Autodesk Inventor part; units mm, degrees
ref_plane "YZ Plane" through (0, 0, 0) normal (1, 0, 0) x (0, 1, 0)
ref_plane "XZ Plane" through (0, 0, 0) normal (0, 1, 0) x (-1, 0, 0)
ref_plane "XY Plane" through (0, 0, 0) normal (0, 0, 1) x (1, 0, 0)
sketch "Sketch1" plane through (0, 0, 0) normal (0, 0, 1) x (1, 0, 0)
  line L0 (0, 12.95) -> (0, -12.95) construction
  line L1 (-21, 0) -> (21, 0) construction
  line L2 (-15, 9.25) -> (15, 9.25)
  line L3 (15, 9.25) -> (15, -9.25)
  line L4 (15, -9.25) -> (-15, -9.25)
  line L5 (-15, -9.25) -> (-15, 9.25)
  point P0 (0, 0)
  dimension "d0" = 18.5
  dimension "d1" = 30
extrude "Extrusion1" add sketch "Sketch1" along normal blind 12
sketch "Sketch2" plane through (0, 0, 0) normal (0, 0, -1) x (-1, 0, 0)
  line L0 (-15, 9.25) -> (15, -9.25) construction
  line L1 (15, 9.25) -> (-15, -9.25) construction
  point P0 (0, 0)
  point P1 (0, 0)
hole "Hole1" at (0, 0, 0) direction (0, 0, 1) diameter 3.242 end through all
sketch "Sketch3" plane through (0, 0, 12) normal (0, 0, 1) x (1, 0, 0)
  line L0 (15, 9.25) -> (15, -9.25)
  line L1 (-15, 9.25) -> (15, 9.25)
  line L2 (-15, -9.25) -> (-15, 9.25)
  line L3 (15, -9.25) -> (-15, -9.25)
  line L4 (-15, 0) -> (15, 0) construction
  line L5 (0, 9.25) -> (0, -9.25) construction
  line L6 (-11.3, 6.3) -> (11.3, 6.3) construction
  line L7 (11.3, 6.3) -> (11.3, -6.3) construction
  line L8 (11.3, -6.3) -> (-11.3, -6.3) construction
  line L9 (-11.3, -6.3) -> (-11.3, 6.3) construction
  dimension "d11" = 12.6
  dimension "d12" = 22.6
hole "Hole2" at (-11.3, 6.3, 12) at (11.3, 6.3, 12) at (11.3, -6.3, 12) at (-11.3, -6.3, 12) direction (0, 0, -1) diameter 3 depth 7
sketch "Sketch4" plane through (0, 0, 12) normal (0, 0, 1) x (1, 0, 0)
  circle A0 centre (11.3, -6.3) radius 1.5
  circle A1 centre (-11.3, 6.3) radius 1.5
  circle A2 centre (0, 0) radius 1.621
  line L0 (-11.3, 6.3) -> (11.3, 6.3)
  line L1 (11.3, 6.3) -> (11.3, -6.3)
  line L2 (11.3, -6.3) -> (-11.3, -6.3)
  line L3 (-11.3, -6.3) -> (-11.3, 6.3)
extrude "Extrusion2" cut sketch "Sketch4" against normal blind 7 contours L1 L2 A0 | A0 L2 L3 A1 L0 L1 | A1 L3 L0 picked at (10.3125, -6.1887) picked at (-10.4586, 5.7713)
sketch "Sketch5" plane through (-15, 9.25, 0) normal (0, 1, 0) x (1, 0, 0)
  line L0 (5.2, -12) -> (5.2, -5) construction
  line L1 (24.8, -12) -> (5.2, -12) construction
  line L2 (24.8, -5) -> (24.8, -12) construction
  line L3 (5.2, -5) -> (24.8, -5) construction
  line L4 (24.8, -8.5) -> (5.2, -8.5) construction
  point P0 (15, 0)
  point P1 (15, -8.5)
  dimension "d33" = 9.8
hole "Hole3" at (0, 9.25, 8.5) direction (0, -1, 0) diameter 2.459 end through all
sketch "Sketch6" plane through (-15, 9.25, 0) normal (0, 1, 0) x (1, 0, 0)
  line L0 (0, 0) -> (30, 0)
  line L1 (15, 2.4) -> (15, -14.4) construction
  line L2 (2.5, 0) -> (27.5, 0)
  line L3 (27.5, 0) -> (27.5, -2)
  line L4 (27.5, -2) -> (2.5, -2)
  line L5 (2.5, -2) -> (2.5, 0)
  point P0 (15, 0)
  dimension "d29" = 25
  dimension "d30" = 2
extrude "Extrusion3" cut sketch "Sketch6" against normal up to next
properties part number "Küvettenklammer_20mm_version3"
Geometry: final body of the model. Coordinates: model frame, mm. A direction names the side the tool comes from. Round coordinates to 2 decimals unless told otherwise and drop trailing zeros. Write each loop counter-clockwise with the first axis right and the second up, starting at its lowest first coordinate (ties: lowest second). Pieces come first, ordered by that corner, then holes.
Item 1: Mould query, pull axis X, two halves, no side actions, for faces 4 (the face through (15, 0, 6)), 5 (the face through (-0.369, -7.796, 9.673)), 6 (the face through (0, -9.25, 7)). Classes: +X half, -X half, draft (parallel to the pull), parting line (faces both ways), or undercut.
Item 2: Material intervals for L1, parallel to Z at x = 0, y = -7.15; L2, parallel to Y at x = 0, z = 3.3; L3, parallel to Y at x = 1.5, z = 10.75, sorted ascending.
Item 3: Section query B-B (y = 0). Return loops of the section in (x, z), plus the area to 3 significant figures.
Item 4: Section query A-A (x = 0). Return loops of the section in (y, z), plus the area to 3 significant figures.
Item 5: Section query C-C (z = 8.5). Return loops of the section in (x, y).
Item 6: Pin query (flat end, axial travel): P1, Ø5, axis at x = 0, y = 0, coming from the -Z side; P2, Ø2, axis at x = 0, z = 8.5, coming from the +Y side; P3, Ø4.5, axis at x = 5.5, y = -1.5, coming from the +Z side. Return the tip coordinate at first contact, or that it passes through.
Item 7: Set-up query: faces 1 (the face through (12.5, 0, 1)), 2 (the face through (1.438, 0.748, 3.521)), 3 (the face through (-11.3, 0, 9)). Return all of +Z, -Z, +X, -X, +Y, -Y with unobstructed straight access to the full face (end or side cutting, diameter ignored); none if empty.
Item 8: Section query D-D (y = -7.5). Return loops of the section in (x, z).
Completed:
1. face 4: +X half
1. face 5: undercut
1. face 6: draft
2. L1: z = 2 to 7.27, 9.73 to 12
2. L2: y = -9.25 to -1.62, 1.62 to 9.25
2. L3: y = -9.25 to -6.3, 6.3 to 9.25
3. outline: (-15, 0) - (-12.5, 0) - (-12.5, 2) - (-1.62, 2) - (-1.62, 5) - (-11.3, 5) - (-11.3, 12) - (-15, 12) - close; (1.62, 2) - (12.5, 2) - (12.5, 0) - (15, 0) - (15, 12) - (11.3, 12) - (11.3, 5) - (1.62, 5) - close
3. area: 142 mm2
4. outline: (-9.25, 2) - (-1.62, 2) - (-1.62, 5) - (-6.3, 5) - (-6.3, 7.27) - (-9.25, 7.27) - close; (-9.25, 9.73) - (-6.3, 9.73) - (-6.3, 12) - (-9.25, 12) - close; (1.62, 2) - (9.25, 2) - (9.25, 7.27) - (6.3, 7.27) - (6.3, 5) - (1.62, 5) - close; (6.3, 9.73) - (9.25, 9.73) - (9.25, 12) - (6.3, 12) - close
4. area: 72.6 mm2
5. outline: (-15, -9.25) - (-1.23, -9.25) - (-1.23, -6.3) - (-9.8, -6.3) arc R1.5 cw (long way) to (-11.3, -4.8) - (-11.3, 4.8) arc R1.5 cw (long way) to (-9.8, 6.3) - (-1.23, 6.3) - (-1.23, 9.25) - (-15, 9.25) - close; (1.23, -9.25) - (15, -9.25) - (15, 9.25) - (1.23, 9.25) - (1.23, 6.3) - (9.8, 6.3) arc R1.5 cw (long way) to (11.3, 4.8) - (11.3, -4.8) arc R1.5 cw (long way) to (9.8, -6.3) - (1.23, -6.3) - close
6. P1: stops at z = 2
6. P2: passes through
6. P3: stops at z = 5
7. face 1: -Z, +Y, -Y
7. face 2: +Z, -Z
7. face 3: +Z
8. outline: (-15, 0) - (-12.5, 0) - (-12.5, 2) - (12.5, 2) - (12.5, 0) - (15, 0) - (15, 12) - (12.2, 12) - (12.2, 5) - (10.4, 5) - (10.4, 12) - (-10.4, 12) - (-10.4, 5) - (-12.2, 5) - (-12.2, 12) - (-15, 12) - close; hole circle Ø2.46 at (0, 8.5)
